Geometry check sheet. Reference: the model listing, model coordinates, mm. A direction names the side the tool comes from. Coordinates: 2 decimals unless noted, no trailing zeros. Put each result on its own line as item: value.
from build123d import *

# Parameters (mm, degrees)
BOSS_EXTRU_1_DEPTH      = 5
ESQUISSE2_R             = 2.75
ENL_V_MAT_EXTRU_1_DEPTH = 213.190951739


with BuildPart() as part:
    # Esquisse1 → Boss.-Extru.1 (new body)
    with BuildSketch(Plane.XY):
        Polygon((112.625631329, 137.374368671), (100, 150), (-100, 150), (-112.625631329, 137.374368671), (-98.483495706, 123.232233047), (-123.232233047, 98.483495706), (-137.374368671, 112.625631329), (-150, 100), (-150, -100), (-137.374368671, -112.625631329), (-123.232233047, -98.483495706), (-98.483495706, -123.232233047), (-112.625631329, -137.374368671), (-100, -150), (100, -150), (112.625631329, -137.374368671), (98.483495706, -123.232233047), (123.232233047, -98.483495706), (137.374368671, -112.625631329), (150, -100), (150, 100), (137.374368671, 112.625631329), (123.232233047, 98.483495706), (98.483495706, 123.232233047), align=None)
    extrude(amount=BOSS_EXTRU_1_DEPTH)

    # Esquisse2 → Enlèv. mat.-Extru.1 (cut, through all)
    with BuildSketch(Plane(origin=(0, 0, 0), x_dir=(-1, 0, 0), z_dir=(0, 0, -1))):
        with Locations((143, -62.5)):
            Circle(ESQUISSE2_R)
        with Locations((143, -94.5)):
            Circle(ESQUISSE2_R)
        with Locations((143, 62.5)):
            Circle(ESQUISSE2_R)
        with Locations((143, 94.5)):
            Circle(ESQUISSE2_R)
        with Locations((-143, -62.5)):
            Circle(ESQUISSE2_R)
        with Locations((-143, -94.5)):
            Circle(ESQUISSE2_R)
        with Locations((-143, 62.5)):
            Circle(ESQUISSE2_R)
        with Locations((-143, 94.5)):
            Circle(ESQUISSE2_R)
    extrude(amount=-ENL_V_MAT_EXTRU_1_DEPTH, mode=Mode.SUBTRACT)


solid = part.part
Q1. Access from +Z, -Z, +X, -X, +Y, -Y to the whole of each face (thin tool, end or side, straight path). Record for faces 4 (the flat face through (110.685, -111.031, 2.465)), 5 (the flat face through (-105.456, -130.204, 2.465)), 6 (the flat face through (105.456, 130.204, 2.465)).
Answer block:
face 4: +Z, -Z
face 5: +Z, -Z, -X
face 6: +Z, -Z, +X
Q2. Depth check by flat-ended pin: pin 1 Ø5 at (x, y) = (-143, 62.5) entering from +Z; pin 2 Ø1.5 at (y, z) = (103, 3) entering from -X. Enter the tip coordinate at first touch or a pass-through.
Answer block:
pin 1: passes through
pin 2: stops at x = -147.75
Q3. Thickness scan on L1, parallel to Y at x = 143, z = 1.3; L2, parallel to Y at x = -114, z = 3.25; L3, parallel to Y at x = 131, z = 3.8. Record the ranges inside material, lowest first. Write a range as [from, to].
Answer block:
L1: y = [-107, -97.25], [-91.75, -65.25], [-59.75, 59.75], [65.25, 91.75], [97.25, 107]
L2: y = [-107.72, 107.72]
L3: y = [-106.25, 106.25]
Q4. Draft check along X on faces 1 (the flat face through (-106, -144, 2)), 2 (the flat face through (144, 106, 2)), 3 (the flat face through (-111.031, -110.685, 2.465)). Enter one of: pulls with the +X half, pulls with the -X half, needs draft (parallel to the pull), parting line crosses it, or undercut.
Answer block:
face 1: pulls with the -X half
face 2: pulls with the +X half
face 3: undercut
Q5. Section check A-A on z = 1.85. State how many separate pieces and enclosed holes the cut face has, then the cut area to 3 significant figures.
Answer block:
separate pieces: 1
enclosed holes: 8
area: 82,000 mm^2
